Can you work these out from the model? Positions are in its coordinate system, mm. A direction names the side the tool comes from. Coordinates: 2 decimals unless noted, no trailing zeros. Order: outer loops, then holes, each group sorted by start corner. A loop starts at its lowest first (then second) coordinate and runs counter-clockwise, first axis right, second up. Notation, with made-up numbers: (28.5, -13) -> (87.5, -13) arc R20 cw to (87.5, 21) -> close; hole circle Ø11 at (77, 26). An arc over 180 degrees is marked (long way). Answer as a JSON object with one key per item and string values. Group by question number.
(1) I want a section at D-D, the plane z = 11.25. List the corners of the cut face in (x, y) for me.
(2) I want a section at C-C, the plane z = 21.25. List the corners of the cut face in (x, y) for me, plus the area to 3 significant figures.
(3) Which directions (+Z, -Z, +X, -X, +Y, -Y) give clear straight access to the entire face, cutting with the end or side of a thin tool? Please do faces 1 (the flat face through (30, 32, 3.556)), 2 (the cylindrical face through (30.133, 1.255, 9.353)), 3 (the flat face through (30, 62, 25.146)).
(4) I want a section at A-A, the plane x = 30.48. List the corners of the cut face in (y, z) for me.
(5) If we mould it in two halves opening along Y, with no side actions, what happens to faces 4 (the flat face through (60.96, 31, 12)), 5 (the flat face through (58.441, 32, 15)), 6 (the flat face through (30, 63.5, 12))? For each: pulls with the +Y half, pulls with the -Y half, needs draft (parallel to the pull), parting line crosses it, or undercut.
(6) I need wall thicknesses on line 1 (X direction, y = 55, z = 12); line 2 (Y direction, x = 11, z = 4.75); line 3 (Y direction, x = 43, z = 16.5). Which ranges of each line are inside material? Lowest first, please.
(7) I want a section at B-B, the plane y = 27. List the corners of the cut face in (x, z) for me, plus the area to 3 significant figures.
(8) For pin 1 (6 mm diameter, centred on x = 52.5, y = 39.5, fed in from +Z), with a flat end and sliding along its axis, tell me the tip position at first contact or that it passes through.
from build123d import *

# Parameters (mm, degrees)
F0_W     = 60.96
F0_H     = 63.5
F1_DEPTH = 25.146
F2_W     = 56.310931
F2_H     = 59.023448
F3_DEPTH = 21.59
F5_DEPTH = 25.4


with BuildPart() as f1:
    # F0 (on Top) → F1 (new body)
    with BuildSketch(Plane.XY):
        with Locations((30.48, 31.75)):
            Rectangle(F0_W, F0_H)
    extrude(amount=F1_DEPTH)

    # F2 (on face) → F3 (cut)
    with BuildSketch(Plane.XY.offset(25.146)):
        with Locations((30.285216, 32.056931)):
            Rectangle(F2_W, F2_H)
    extrude(amount=-F3_DEPTH, mode=Mode.SUBTRACT)

    # F4 (on face) → F5 (cut)
    with BuildSketch(Plane.XZ):
        with BuildLine():
            ThreePointArc((14.683233, 25.146), (30.48, 9.349233), (46.276767, 25.146))
            Line((46.276767, 25.146), (14.683233, 25.146))
        make_face()
    extrude(amount=-F5_DEPTH, mode=Mode.SUBTRACT)


solid = f1.part
Computed values:
{
 "1": {"outline": "(0, 0) -> (22.97, 0) -> (22.97, 2.55) -> (2.13, 2.55) -> (2.13, 61.57) -> (58.44, 61.57) -> (58.44, 2.55) -> (37.99, 2.55) -> (37.99, 0) -> (60.96, 0) -> (60.96, 63.5) -> (0, 63.5) -> close"},
 "2": {"outline": "(0, 0) -> (15.17, 0) -> (15.17, 2.55) -> (2.13, 2.55) -> (2.13, 61.57) -> (58.44, 61.57) -> (58.44, 2.55) -> (45.79, 2.55) -> (45.79, 0) -> (60.96, 0) -> (60.96, 63.5) -> (0, 63.5) -> close", "area": "469 mm2"},
 "3": {"face 1": "+Z", "face 2": "+Z, -Y", "face 3": "+Z, +X, -X, +Y, -Y"},
 "4": {"outline": "(0, 0) -> (63.5, 0) -> (63.5, 25.15) -> (61.57, 25.15) -> (61.57, 3.56) -> (2.55, 3.56) -> (2.55, 9.35) -> (0, 9.35) -> close"},
 "5": {"face 4": "needs draft", "face 5": "undercut", "face 6": "pulls with the +Y half"},
 "6": {"line 1": "x = 0 to 2.13, 58.44 to 60.96", "line 2": "y = 0 to 2.55, 61.57 to 63.5", "line 3": "y = 61.57 to 63.5"},
 "7": {"outline": "(0, 0) -> (60.96, 0) -> (60.96, 25.15) -> (58.44, 25.15) -> (58.44, 3.56) -> (2.13, 3.56) -> (2.13, 25.15) -> (0, 25.15) -> close", "area": "317 mm2"},
 "8": {"pin 1": "stops at z = 3.56"}
}
